Geometry check sheet. Reference: the model listing, model coordinates, mm. Round coordinates to 2 decimals unless told otherwise and drop trailing zeros. Loops run counter-clockwise (first coordinate to the right, second up) from the corner with the lowest first, then second, coordinate; pieces in that order, holes last. Notation, with made-up numbers: (48.5, -37.5) -> (52.5, -37.5) arc R29 ccw to (52.5, -16.5) -> close; hole circle Ø7 at (10, 42.5). An arc over 180 degrees is marked (long way). Use a Markdown table: item, result. Add a question column.
Q1. Material ranges on L1, parallel to Y at x = -479, z = 111.5; L2, parallel to Y at x = 64, z = -15, recorded low to high.
Q2. Sectioned sample at C-C, the plane x = -34.5. Enter the section's corners in (y, z).
Q3. Sectioned sample at D-D, the plane x = -500. Enter the section's corners in (y, z).
Q4. Sectioned sample at B-B, the plane z = -182.5. Enter the section's corners in (x, y), then the cut area to 3 significant figures.
Q5. Gauge pin test, flat ends, axial feed: P1, Ø5, axis at x = 290.5, z = 330, coming from the -Y side; P2, Ø10, axis at x = -283, z = 426.5, coming from the +Y side; P3, Ø7.5, axis at y = 12, z = -124.5, coming from the -X side. Record the tip position at first contact, or that the pin passes through.
Q6. Sectioned sample at A-A, the plane y = -521.5. Enter the section's corners in (x, z), then the cut area to 3 significant figures.
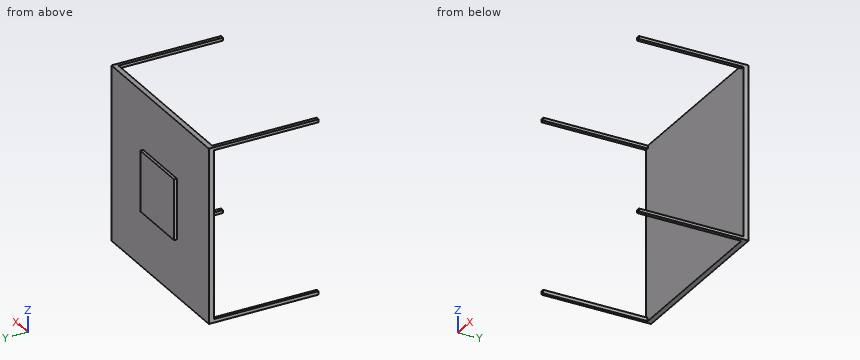
```python
from build123d import *

# Parameters (mm, degrees)
SKETCH1_W           = 520
SKETCH1_H           = 520
BOSS_EXTRUDE1_DEPTH = 25
SKETCH2_W           = 1500
SKETCH2_H           = 1500
BOSS_EXTRUDE2_DEPTH = 45
SKETCH3_W           = 30
SKETCH3_H           = 25
BOSS_EXTRUDE3_DEPTH = 900
SKETCH4_W           = 30
SKETCH4_H           = 25
BOSS_EXTRUDE4_DEPTH = 900
SKETCH5_W           = 30
SKETCH5_H           = 25
BOSS_EXTRUDE5_DEPTH = 900
SKETCH6_W           = 25
SKETCH6_H           = 30
BOSS_EXTRUDE6_DEPTH = 900


with BuildPart() as part:
    # Sketch1 → Boss-Extrude1 (new body)
    with BuildSketch(Plane(origin=(0, 0, 0), x_dir=(1, 0, 0), z_dir=(0, 1, 0))):
        Rectangle(SKETCH1_W, SKETCH1_H)
    extrude(amount=BOSS_EXTRUDE1_DEPTH)

    # Sketch2 → Boss-Extrude2 (add)
    with BuildSketch(Plane.XZ):
        Rectangle(SKETCH2_W, SKETCH2_H)
    extrude(amount=BOSS_EXTRUDE2_DEPTH)

    # Sketch3 → Boss-Extrude3 (add)
    with BuildSketch(Plane.XZ.offset(45)):
        with Locations((735, 737.5)):
            Rectangle(SKETCH3_W, SKETCH3_H)
    extrude(amount=BOSS_EXTRUDE3_DEPTH)

    # Sketch4 → Boss-Extrude4 (add)
    with BuildSketch(Plane.XZ.offset(45)):
        with Locations((-735, 737.5)):
            Rectangle(SKETCH4_W, SKETCH4_H)
    extrude(amount=BOSS_EXTRUDE4_DEPTH)

    # Sketch5 → Boss-Extrude5 (add)
    with BuildSketch(Plane.XZ.offset(45)):
        with Locations((735, -737.5)):
            Rectangle(SKETCH5_W, SKETCH5_H)
    extrude(amount=BOSS_EXTRUDE5_DEPTH)

    # Sketch6 → Boss-Extrude6 (add)
    with BuildSketch(Plane.XZ.offset(45)):
        with Locations((-737.5, -735)):
            Rectangle(SKETCH6_W, SKETCH6_H)
    extrude(amount=BOSS_EXTRUDE6_DEPTH)


solid = part.part
```
Values:
| question | item | result |
|---|---|---|
| 1 | L1 | -45 to 0 |
| 1 | L2 | -45 to 25 |
| 2 | outline | (-45, -750) -> (0, -750) -> (0, -260) -> (25, -260) -> (25, 260) -> (0, 260) -> (0, 750) -> (-45, 750) -> close |
| 3 | outline | (-45, -750) -> (0, -750) -> (0, 750) -> (-45, 750) -> close |
| 4 | outline | (-750, -45) -> (750, -45) -> (750, 0) -> (260, 0) -> (260, 25) -> (-260, 25) -> (-260, 0) -> (-750, 0) -> close |
| 4 | area | 80,500 mm^2 |
| 5 | P1 | y = -45 |
| 5 | P2 | y = 0 |
| 5 | P3 | x = -260 |
| 6 | outline | (-750, -750) -> (-725, -750) -> (-725, -720) -> (-750, -720) -> close; (-750, 725) -> (-720, 725) -> (-720, 750) -> (-750, 750) -> close; (720, -750) -> (750, -750) -> (750, -725) -> (720, -725) -> close; (720, 725) -> (750, 725) -> (750, 750) -> (720, 750) -> close |
| 6 | area | 3,000 mm^2 |
